Geometry: final body of the model. Coordinates: model frame, mm. Round coordinates to 2 decimals unless told otherwise and drop trailing zeros. Loops run counter-clockwise (first coordinate to the right, second up) from the corner with the lowest first, then second, coordinate; pieces in that order, holes last. Notation, with made-up numbers: M 21.5,38 L 73.5,38 A10 ccw 73.5,46 Z; hole C 19,88.5 d10. An arc over 180 degrees is marked long. Answer as a JSON object with one key per item and string values.
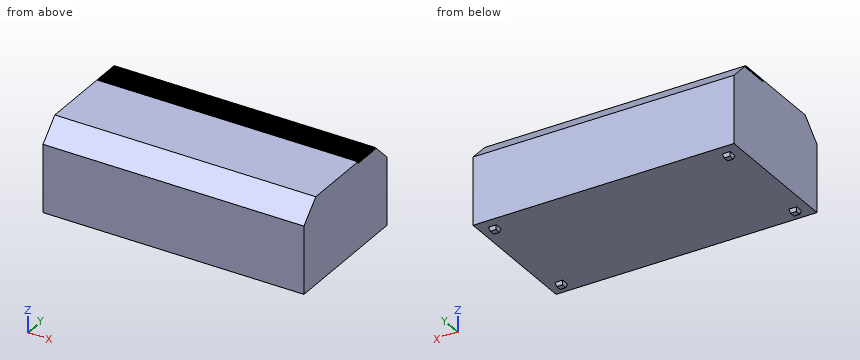
```python
from build123d import *

# Parameters (mm, degrees)
F0_W     = 270
F0_H     = 140
F1_DEPTH = 90
F2_SIZE  = 20
F3_W     = 1
F3_H     = 2
F4_DEPTH = 270
F5_W     = 8
F5_H     = 8
F6_DEPTH = 4
F6_TAPER = 15


with BuildPart() as f1:
    # F0 (on Top) → F1 (new body)
    with BuildSketch(Plane.XY):
        Rectangle(F0_W, F0_H)
    extrude(amount=F1_DEPTH)

    # F2
    f2_edges = [f1.edges().sort_by_distance(p)[0] for p in [
        (0, -70, 90),
        (0, 70, 90),
    ]]
    chamfer(f2_edges, length=F2_SIZE)

    # F3 (on face) → F4 (cut, through all)
    with BuildSketch(Plane.YZ.offset(135)):
        with Locations((21.4087878466, 89)):
            Rectangle(F3_W, F3_H)
        with Locations((23.4087878466, 89)):
            Rectangle(F3_W, F3_H)
        with Locations((25.4087878466, 89)):
            Rectangle(F3_W, F3_H)
        with Locations((27.4087878466, 89)):
            Rectangle(F3_W, F3_H)
        with Locations((29.4087878466, 89)):
            Rectangle(F3_W, F3_H)
        with Locations((31.4087878466, 89)):
            Rectangle(F3_W, F3_H)
        with Locations((33.4087878466, 89)):
            Rectangle(F3_W, F3_H)
        with Locations((35.4087878466, 89)):
            Rectangle(F3_W, F3_H)
        with Locations((37.4087878466, 89)):
            Rectangle(F3_W, F3_H)
        with Locations((39.4087878466, 89)):
            Rectangle(F3_W, F3_H)
        with Locations((41.4087878466, 89)):
            Rectangle(F3_W, F3_H)
        with Locations((43.4087878466, 89)):
            Rectangle(F3_W, F3_H)
        with Locations((45.4087878466, 89)):
            Rectangle(F3_W, F3_H)
        with Locations((47.4087878466, 89)):
            Rectangle(F3_W, F3_H)
        with Locations((49.4087878466, 89)):
            Rectangle(F3_W, F3_H)
    extrude(amount=-F4_DEPTH, mode=Mode.SUBTRACT)

    # F5 (on face) → F6 (join)
    with BuildSketch(Plane(origin=(0, 0, 0), x_dir=(1, 0, 0), z_dir=(0, 0, -1))):
        with Locations((121, 56)):
            Rectangle(F5_W, F5_H)
        with Locations((121, -56)):
            Rectangle(F5_W, F5_H)
        with Locations((-121, 56)):
            Rectangle(F5_W, F5_H)
        with Locations((-121, -56)):
            Rectangle(F5_W, F5_H)
    extrude(amount=F6_DEPTH, taper=F6_TAPER)


solid = f1.part
```
1) Line query: probe 1 along Z at (x, y) = (-94.5, -20); probe 2 along Z at (x, y) = (-94.5, 23); probe 3 along Y at (x, z) = (14, 77.5). Output: solid intervals per line, ascending.
Geometry results:
{"probe 1": "0 to 90", "probe 2": "0 to 88", "probe 3": "-62.5 to 62.5"}
2) Cut plane A-A on z = 75. Return the cut outline in (x, y), and give its area (3 significant figures).
Geometry results:
{"outline": "M -135,-65 L 135,-65 L 135,65 L -135,65 Z", "area": "35,100 mm2"}
3) Cut plane B-B on y = 3.5. Return the cut outline in (x, z), and give its area (3 significant figures).
Geometry results:
{"outline": "M -135,0 L 135,0 L 135,90 L -135,90 Z", "area": "24,300 mm2"}
4) First-contact query: pin 1 (1.6 mm diameter, centred on x = 49, z = 89, fed in from -Y); pin 2 (0.5 mm diameter, centred on x = -14.5, y = 43, fed in from +Z); pin 3 (2 mm diameter, centred on x = 33.5, z = 88.5, fed in from +Y); pin 4 (0.6 mm diameter, centred on x = -53, z = 89, fed in from -Y). Flat tips, straight axial feed; report the tip coordinate or a pass-through.
Geometry results:
{"pin 1": "y = -51.8", "pin 2": "z = 90", "pin 3": "y = 52.5", "pin 4": "y = -51.3"}
